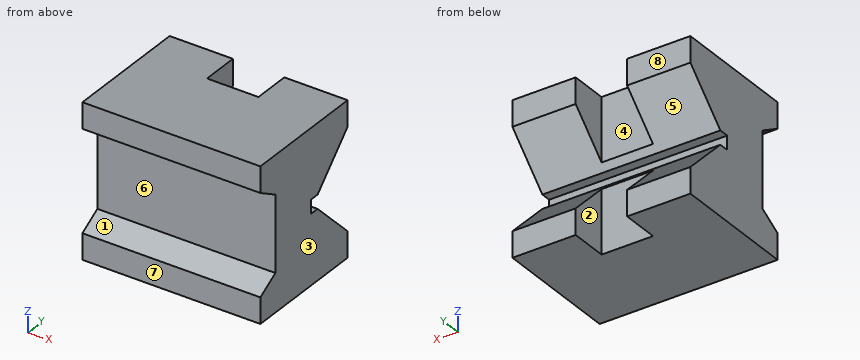
```python
from build123d import *

# Parameters (mm, degrees)
IZIM6_W                     = 900
IZIM6_H                     = 640
Y_KSEKLIK_EKSTR_ZYON3_DEPTH = 770
IZIM7_W                     = 260
IZIM7_H                     = 190
KES_EKSTR_ZYON4_DEPTH       = 770
KES_EKSTR_ZYON6_REACH       = 1228.907
KES_EKSTR_ZYON7_DEPTH       = 900


with BuildPart() as part:
    # Çizim6 → Yükseklik-Ekstrüzyon3 (new body)
    with BuildSketch(Plane.XY):
        Rectangle(IZIM6_W, IZIM6_H)
    extrude(amount=Y_KSEKLIK_EKSTR_ZYON3_DEPTH)

    # Çizim7 → Kes-Ekstrüzyon4 (cut)
    with BuildSketch(Plane.XY.offset(770)):
        with Locations((0, 225)):
            Rectangle(IZIM7_W, IZIM7_H)
    extrude(amount=-KES_EKSTR_ZYON4_DEPTH, mode=Mode.SUBTRACT)

    # Kes-Ekstrüzyon6: up to this face of the body (flat: up to its plane)
    kes_ekstr_zyon6_end = Plane(part.part.faces().sort_by_distance((-450, 0, 385))[0])
    # Çizim8 → Kes-Ekstrüzyon6 (cut, up to the picked face)
    with BuildSketch(Plane(origin=(450, 0, 0), x_dir=(0, 0, -1), z_dir=(1, 0, 0)), mode=Mode.PRIVATE) as kes_ekstr_zyon6_sk1:
        Polygon((-350, 50), (-350, 100), (-130, 320), (-640, 320), (-420, 100), (-420, 50), align=None)
    kes_ekstr_zyon6_tool1 = split(extrude(kes_ekstr_zyon6_sk1.sketch, amount=-KES_EKSTR_ZYON6_REACH, mode=Mode.PRIVATE), bisect_by=kes_ekstr_zyon6_end, keep=Keep.BOTH, mode=Mode.PRIVATE)
    add(kes_ekstr_zyon6_tool1.solids().sort_by(Axis((450, 229.348687, 385), (-1, 0, 0)))[0], mode=Mode.SUBTRACT)

    # Çizim13 → Kes-Ekstrüzyon7 (cut)
    with BuildSketch(Plane(origin=(450, 0, 0), x_dir=(0, 0, -1), z_dir=(1, 0, 0))):
        Polygon((-640, -320), (-576.491470389, -210), (-193.508529611, -210), (-130, -320), align=None)
    extrude(amount=-KES_EKSTR_ZYON7_DEPTH, mode=Mode.SUBTRACT)


solid = part.part
```
Here's how the part is built. I have some questions about the finished solid (model axes, mm). Face numbers are marked on the shaded views. A direction names the side the tool comes from. Coordinates: 2 decimals unless noted, no trailing zeros. Order: outer loops, then holes, each group sorted by start corner. A loop starts at its lowest first (then second) coordinate and runs counter-clockwise, first axis right, second up. Notation, with made-up numbers: (9.25, 15) - (14.25, 15) arc R7 ccw to (14.25, 25) - close; hole circle Ø1 at (63.5, -21). An arc over 180 degrees is marked (long way). One line per question, with ' | ' between items.
(1) Suppose I cut it at C-C on z = 272.5. List the corners of the cut face in (x, y) for me, and give its area (3 significant figures).
Report:
outline: (-450, -210) - (450, -210) - (450, 177.5) - (130, 177.5) - (130, 130) - (-130, 130) - (-130, 177.5) - (-450, 177.5) - close | area: 336,000 mm2
(2) Will these pins go through, and if not, where does the flat tip stop? pin 1 (1.5 mm diameter, centred on x = 226.5, z = 501.5, fed in from -Y); pin 2 (10 mm diameter, centred on x = 133, z = 205.5, fed in from +Y).
Report:
pin 1: stops at y = -210 | pin 2: stops at y = 249.5
(3) If I drill on L1, parallel to X at y = 226.5, z = 107; L2, parallel to Z at x = 364, y = 63.5; L3, parallel to Y at x = -81.5, z = 452.5, over which ranges is the centre line in solid material (lowest first)?
Report:
L1: x = -450 to -130, 130 to 450 | L2: z = 0 to 350, 420 to 770 | L3: y = -210 to 130
(4) If we mould it in two halves opening along X, with no side actions, what happens to the marked faces 1, 2 and 3? For each: pulls with the +X half, pulls with the -X half, needs draft (parallel to the pull), parting line crosses it, or undercut.
Report:
face 1: needs draft | face 2: undercut | face 3: pulls with the +X half
(5) For the marked faces 4, 5, 6, 7 and 8, which set-ups out of +Z, -Z, +X, -X, +Y, -Y let a thin tool reach every point of the face, with its end or its side?
Report:
face 4: +Z, -Z, +Y | face 5: +X, -X, +Y | face 6: +X, -X, -Y | face 7: +Z, -Z, +X, -X, -Y | face 8: +Z, -Z, +X, -X, +Y
(6) Suppose I cut it at B-B on x = 12.5. List the corners of the cut face in (y, z) for me, and give its area (3 significant figures).
Report:
outline: (-320, 0) - (130, 0) - (130, 320) - (100, 350) - (50, 350) - (50, 420) - (100, 420) - (130, 450) - (130, 770) - (-320, 770) - (-320, 640) - (-210, 576.49) - (-210, 193.51) - (-320, 130) - close | area: 291,000 mm2
(7) Suppose I cut it at A-A on y = 217. List the corners of the cut face in (x, z) for me, and give its area (3 significant figures).
Report:
outline: (-450, 0) - (-130, 0) - (-130, 233) - (-450, 233) - close; (-450, 537) - (-130, 537) - (-130, 770) - (-450, 770) - close; (130, 0) - (450, 0) - (450, 233) - (130, 233) - close; (130, 537) - (450, 537) - (450, 770) - (130, 770) - close | area: 298,000 mm2
(8) Suppose I cut it at D-D on z = 87. List the corners of the cut face in (x, y) for me, and give its area (3 significant figures).
Report:
outline: (-450, -320) - (450, -320) - (450, 320) - (130, 320) - (130, 130) - (-130, 130) - (-130, 320) - (-450, 320) - close | area: 527,000 mm2
